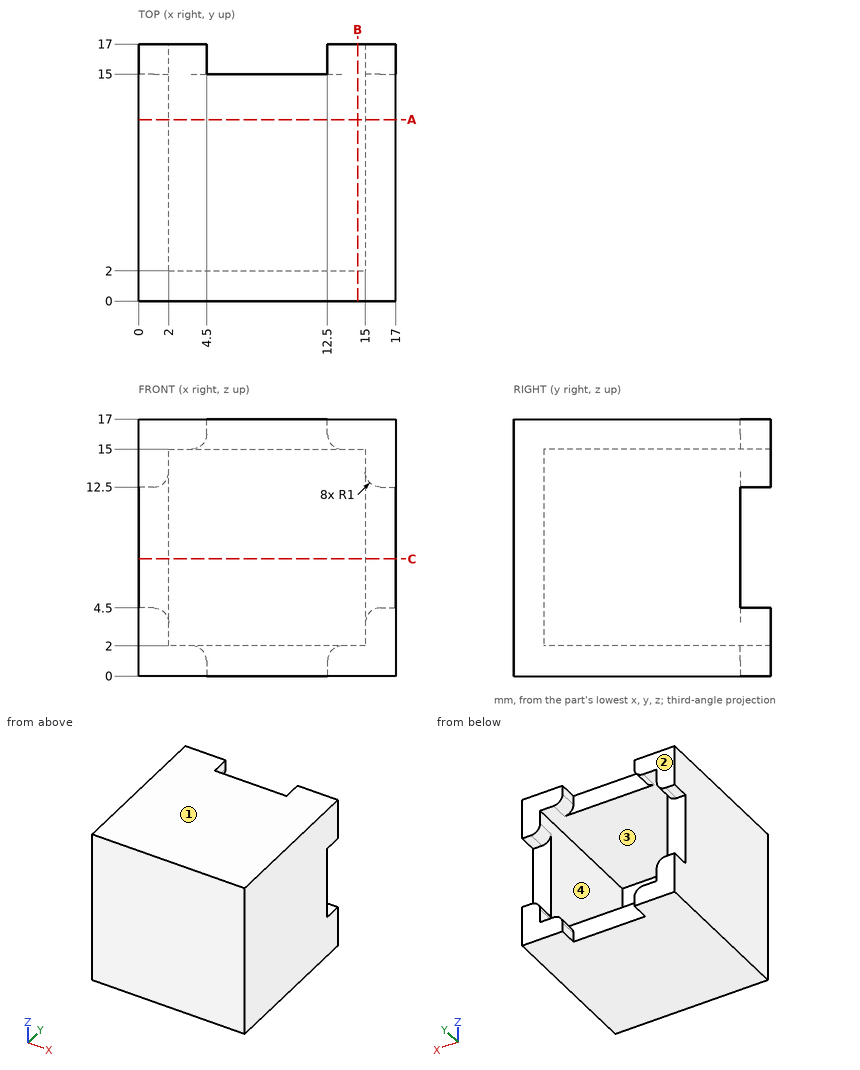
Drawing for the job (mm, zero at the part's lowest x, y, z). Round coordinates to 2 decimals unless told otherwise and drop trailing zeros. Write each loop counter-clockwise with the first axis right and the second up, starting at its lowest first coordinate (ties: lowest second). Pieces come first, ordered by that corner, then holes. Notation, with made-up numbers: (87, 79) - (133, 79) arc R33 ccw to (133, 108) - close; hole circle Ø5 at (45.5, 14.5). An arc over 180 degrees is marked (long way). Return JSON: item names as keys, results as strings. Group by question number.
Item 1: Mould opens along Z. For the marked faces 1, 2, 3 and 4 say: +Z half, -Z half, draft (parallel to the pull), parting line (faces both ways), or undercut.
Item 2: Band-saw the part on C-C on z = 7.75. List the corners of the cut face in (x, y).
Item 3: Probe probe 1 along Z at (x, y) = (12.5, 8); probe 2 along Z at (x, y) = (16.25, 15.75). List the from-to ranges inside material, lowest first.
Item 4: Band-saw the part on B-B on x = 14.5. List the corners of the cut face in (y, z), plus the area to 3 significant figures.
Item 5: Flat gauge pins, fed straight in: pin 1 Ø2 at (x, z) = (11, 0.5) entering from +Y; pin 2 Ø1.5 at (x, z) = (13, 14) entering from +Y. Where does each tip first touch, or does it go through?
Item 6: Band-saw the part on A-A on y = 12. List the corners of the cut face in (x, z).
Resolved:
{
 "1": {"face 1": "+Z half", "face 2": "draft", "face 3": "undercut", "face 4": "undercut"},
 "2": {"outline": "(0, 0) - (17, 0) - (17, 15) - (15, 15) - (15, 2) - (2, 2) - (2, 15) - (0, 15) - close"},
 "3": {"probe 1": "z = 0 to 2, 15 to 17", "probe 2": "z = 0 to 4.5, 12.5 to 17"},
 "4": {"outline": "(0, 0) - (17, 0) - (17, 2) - (2, 2) - (2, 15) - (17, 15) - (17, 17) - (0, 17) - close", "area": "94.0 mm²"},
 "5": {"pin 1": "stops at y = 15", "pin 2": "stops at y = 2"},
 "6": {"outline": "(0, 0) - (17, 0) - (17, 17) - (0, 17) - close; hole (2, 2) - (15, 2) - (15, 15) - (2, 15) - close"}
}
